Part model, mm, in its own coordinate system. Round coordinates to 2 decimals unless told otherwise and drop trailing zeros. Write each loop counter-clockwise with the first axis right and the second up, starting at its lowest first coordinate (ties: lowest second). Pieces come first, ordered by that corner, then holes. Notation, with made-up numbers: M 45.25,-1 L 72.25,-1 A25 ccw 72.25,15 Z; hole C -26,87 d8. An arc over 180 degrees is marked long. Answer as a JSON object with one key per item and string values. Group by question number.
1. Band-saw the part on C-C, the plane z = -23.5. Write the cut outline in (x, y).
2. Band-saw the part on B-B, the plane x = 0. Write the cut outline in (y, z).
3. Drop flat-ended pins along their axis: pin 1 (2.5 mm diameter, centred on x = 0, z = 3.3, fed in from -Y); pin 2 (4 mm diameter, centred on x = -50, z = 28.5, fed in from +Y). Give the stop position or say it passes through.
4. Band-saw the part on A-A, the plane z = -13.5. Write the cut outline in (x, y).
5. Drill centre lines: line 1 (X direction, y = 0.6, z = -13.5); line 2 (X direction, y = 2.05, z = 3.3); line 3 (X direction, y = 0.25, z = 29). Where is each one in solid material? Low to high. Write a range as from..to.
6. Band-saw the part on D-D, the plane x = 50. Write the cut outline in (y, z), plus the area to 3 significant figures.
from build123d import *

# Parameters (mm, degrees)
BOSS_EXTRUDE1_DEPTH = 4
SKETCH4_R           = 1.7
CUT_EXTRUDE1_DEPTH  = 4
CHAMFER1_SIZE       = 1.65


with BuildPart() as part:
    # Sketch1 → Boss-Extrude1 (new body)
    with BuildSketch(Plane(origin=(0, 0, 0), x_dir=(1, 0, 0), z_dir=(0, 1, 0))):
        with BuildLine():
            Line((-74, 43.5), (-74, 49.7434598))
            ThreePointArc((-74, 49.7434598), (-50, 43.5), (-26, 49.7434598))
            Line((-26, 49.7434598), (26, 49.7434598))
            ThreePointArc((26, 49.7434598), (50, 43.5), (74, 49.7434598))
            Line((74, 49.7434598), (74, 43.5))
            Line((74, 43.5), (74, -43.5))
            Line((74, -43.5), (-74, -43.5))
            Line((-74, -43.5), (-74, 43.5))
        make_face()
    extrude(amount=BOSS_EXTRUDE1_DEPTH)

    # Sketch4 → Cut-Extrude1 (cut)
    with BuildSketch(Plane(origin=(0, 4, 0), x_dir=(1, 0, 0), z_dir=(0, 1, 0))):
        with Locations(Location((-50, -28.5, 0), (0, 0, 270))):
            Circle(SKETCH4_R)
        with Locations(Location((-50, 13.5, 0), (0, 0, 270))):
            Circle(SKETCH4_R)
        with Locations(Location((0, -3.3, 0), (0, 0, 270))):
            Circle(SKETCH4_R)
        with Locations(Location((0, 23.5, 0), (0, 0, 270))):
            Circle(SKETCH4_R)
        with Locations(Location((50, -28.5, 0), (0, 0, 270))):
            Circle(SKETCH4_R)
        with Locations(Location((50, 13.5, 0), (0, 0, 270))):
            Circle(SKETCH4_R)
    extrude(amount=-CUT_EXTRUDE1_DEPTH, mode=Mode.SUBTRACT)

    # Chamfer1
    chamfer1_edges = [part.edges().sort_by_distance(p)[0] for p in [
        (50, 4, 26.8),
        (0, 4, -25.2),
        (0, 4, 1.6),
        (0, 0, 1.6),
        (-50, 4, -15.2),
        (50, 4, -15.2),
        (-50, 4, 26.8),
    ]]
    chamfer(chamfer1_edges, length=CHAMFER1_SIZE)


solid = part.part
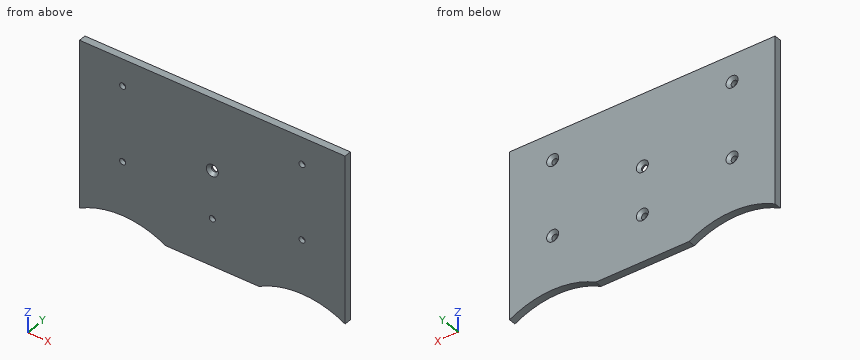
Worked answers:
{
 "1": {"outline": "M -74,0 L -1.7,0 L -1.7,2.35 L -3.35,4 L -74,4 Z; M 1.7,0 L 74,0 L 74,4 L 3.35,4 L 1.7,2.35 Z"},
 "2": {"outline": "M 0,-49.74 L 4,-49.74 L 4,-26.85 L 2.35,-25.2 L 0,-25.2 Z; M 0,-21.8 L 2.35,-21.8 L 4,-20.15 L 4,-0.05 L 2.35,1.6 L 1.65,1.6 L 0,-0.05 Z; M 0,6.65 L 1.65,5 L 2.35,5 L 4,6.65 L 4,43.5 L 0,43.5 Z"},
 "3": {"pin 1": "passes through", "pin 2": "stops at y = 2.65"},
 "4": {"outline": "M -74,0 L -51.7,0 L -51.7,2.35 L -53.35,4 L -74,4 Z; M -48.3,0 L 48.3,0 L 48.3,2.35 L 46.65,4 L -46.65,4 L -48.3,2.35 Z; M 51.7,0 L 74,0 L 74,4 L 53.35,4 L 51.7,2.35 Z"},
 "5": {"line 1": "x = -74..-51.7, -48.3..48.3, 51.7..74", "line 2": "x = -74..-1.7, 1.7..74", "line 3": "x = -74..-51.62, -48.38..48.38, 51.62..74"},
 "6": {"outline": "M 0,-43.5 L 4,-43.5 L 4,-16.85 L 2.35,-15.2 L 0,-15.2 Z; M 0,-11.8 L 2.35,-11.8 L 4,-10.15 L 4,25.15 L 2.35,26.8 L 0,26.8 Z; M 0,30.2 L 2.35,30.2 L 4,31.85 L 4,43.5 L 0,43.5 Z", "area": "315 mm^2"}
}
